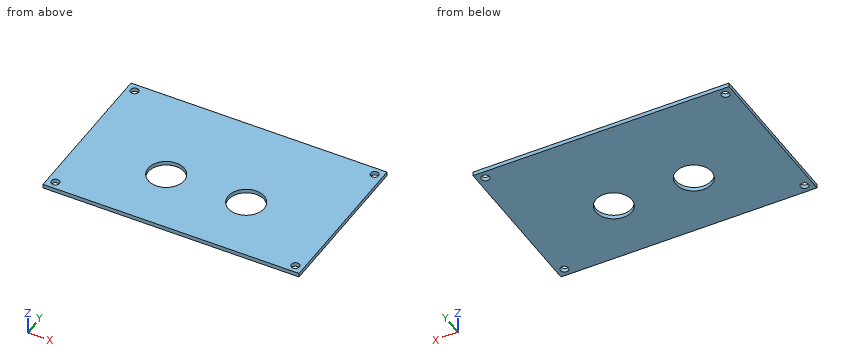
Autodesk Inventor part; units mm, degrees
ref_plane "Work Plane1" through (-101.6, 0, 0) normal (1, 0, 0) x (0, 0, -1)
ref_plane "YZ Plane" through (0, 0, 0) normal (1, 0, 0) x (0, 1, 0)
ref_plane "XZ Plane" through (0, 0, 0) normal (0, 1, 0) x (-1, 0, 0)
sketch "Sketch1" plane through (0, 0, 0) normal (0, 0, 1) x (1, 0, 0)
  line L0 (0, 0) -> (-203.2, 0)
  line L1 (-203.2, 0) -> (-203.2, 127)
  line L2 (-203.2, 127) -> (0, 127)
  line L3 (0, 127) -> (0, 0)
  dimension "d0" = 127
  dimension "d1" = 203.2
extrude "Extrusion1" add sketch "Sketch1" along normal blind 3.175
sketch "Sketch2" plane through (0, 0, 3.175) normal (0, 0, 1) x (1, 0, 0)
  circle A0 centre (-69.85, 50.8) radius 14.2875
  line L0 (0, 0) -> (0, 127)
  line L1 (-203.2, 0) -> (0, 0)
  circle A1 centre (-133.35, 50.8) radius 14.2875
  line L2 (-101.6, 0) -> (-101.6, 50.8)
  line L3 (-101.6, 50.8) -> (-69.85, 50.8)
  line L4 (-69.85, 50.8) -> (-133.35, 50.8)
  dimension "d4" = 28.575
  dimension "d8" = 28.575
  dimension "d9" = 50.8
  dimension "d28" = 63.5
  dimension "d29" = 31.75
extrude "Extrusion2" cut sketch "Sketch2" against normal blind 3.175
sketch "Sketch3" plane through (0, 0, 3.175) normal (0, 0, 1) x (1, 0, 0)
  circle A0 centre (-6.35, 6.35) radius 3.175
  line L0 (0, 0) -> (0, 127)
  line L1 (-203.2, 0) -> (0, 0)
  circle A1 centre (-6.35, 120.65) radius 3.175
  line L2 (0, 127) -> (-203.2, 127)
  circle A2 centre (-196.85, 120.65) radius 3.175
  circle A3 centre (-196.85, 6.35) radius 3.175
  line L3 (-203.2, 127) -> (-203.2, 0)
  dimension "d12" = 6.35
  dimension "d13" = 6.35
  dimension "d14" = 6.35
  dimension "d15" = 6.35
  dimension "d16" = 6.35
  dimension "d17" = 6.35
  dimension "d18" = 6.35
  dimension "d19" = 6.35
  dimension "d20" = 6.35
  dimension "d30" = 6.35
  dimension "d31" = 6.35
  dimension "d32" = 6.35
hole "Hole1" at (-196.85, 120.65, 3.175) at (-196.85, 6.35, 3.175) at (-6.35, 6.35, 3.175) at (-6.35, 120.65, 3.175) direction (0, 0, -1) diameter 6.35 end through all
ref_plane "Work Plane1" through (-101.6, 0, 0) normal (1, 0, 0) x (0, 0, -1)
equation "\"d29\" = 0.5 * d28"
properties part number "Gearbox plate with motor"
For this review, take the finished solid that the model builds, in its own axes (mm). Round coordinates to 2 decimals unless told otherwise and drop trailing zeros. Order: outer loops, then holes, each group sorted by start corner. A loop starts at its lowest first (then second) coordinate and runs counter-clockwise, first axis right, second up. Notation, with made-up numbers: (46, -22.75) -> (92, -22.75) arc R28 cw to (92, 8.25) -> close; hole circle Ø1 at (-37.75, 89.25). An arc over 180 degrees is marked (long way). Use a Markdown table: item, result.
Item 1: Take a section at A-A (y = 50.8). State the section outline as (x, z) points (1 decimal), plus the area to 3 significant figures.
Resolved:
| item | result |
|---|---|
| outline | (-203.2, 0) -> (-147.6, 0) -> (-147.6, 3.2) -> (-203.2, 3.2) -> close; (-119.1, 0) -> (-84.1, 0) -> (-84.1, 3.2) -> (-119.1, 3.2) -> close; (-55.6, 0) -> (0, 0) -> (0, 3.2) -> (-55.6, 3.2) -> close |
| area | 464 mm² |
Item 2: Take a section at B-B (x = -196.85). State the section outline as (y, z) points (3 decimals), plus the area to 3 significant figures.
Resolved:
| item | result |
|---|---|
| outline | (0, 0) -> (3.175, 0) -> (3.175, 3.175) -> (0, 3.175) -> close; (9.525, 0) -> (117.475, 0) -> (117.475, 3.175) -> (9.525, 3.175) -> close; (123.825, 0) -> (127, 0) -> (127, 3.175) -> (123.825, 3.175) -> close |
| area | 363 mm² |
Item 3: Take a section at C-C (x = -69.85). State the section outline as (y, z) points (1 decimal), plus the area to 4 significant figures.
Resolved:
| item | result |
|---|---|
| outline | (0, 0) -> (36.5, 0) -> (36.5, 3.2) -> (0, 3.2) -> close; (65.1, 0) -> (127, 0) -> (127, 3.2) -> (65.1, 3.2) -> close |
| area | 312.5 mm² |
Item 4: For line 1 along Y through (x, z) = (-6.35, 0.75) (3 decimals); line 2 along X through (y, z) = (120.65, 0.7) (3 decimals); line 3 along Y through (x, z) = (-138.5, 2.2), list the stretches that pass through material, from the lowest coordinate up. Write a range as [from, to].
Resolved:
| item | result |
|---|---|
| line 1 | y = [0, 3.175], [9.525, 117.475], [123.825, 127] |
| line 2 | x = [-203.2, -200.025], [-193.675, -9.525], [-3.175, 0] |
| line 3 | y = [0, 37.47], [64.13, 127] |
Item 5: Take a section at D-D (z = 1.8). State how many separate pieces and enclosed holes the cut face has, plus the area to 3 significant figures.
Resolved:
| item | result |
|---|---|
| separate pieces | 1 |
| enclosed holes | 6 |
| area | 24,400 mm² |
